Input: part model. Units: mm. Frame: model coordinates. Coordinates: 2 decimals unless noted, no trailing zeros. Order: outer loops, then holes, each group sorted by start corner. A loop starts at its lowest first (then second) coordinate and runs counter-clockwise, first axis right, second up. Notation, with made-up numbers: (-11, 17) -> (5, 17) arc R31 cw to (5, 44) -> close; hole circle Ø9 at (-18.5, 11). An arc over 180 degrees is marked (long way). Write each question's results on one line, items separated by ' | '.
```python
from build123d import *

# Parameters (mm, degrees)
SKETCH1_W                   = 80
SKETCH1_H                   = 130
SKETCH1_R                   = 3.5
BOSS_EXTRUDE1_DEPTH         = 8
DODANIE_WYCI_GNI_CIE1_DEPTH = 6
SZKIC2_W                    = 2
SZKIC2_H                    = 6
WYTNIJ_WYCI_GNI_CIE1_DEPTH  = 40


with BuildPart() as part:
    # Sketch1 → Boss-Extrude1 (new body)
    with BuildSketch(Plane(origin=(0, 0, 0), x_dir=(0, -1, 0), z_dir=(-1, 0, 0))):
        with Locations((-35, 60)):
            Rectangle(SKETCH1_W, SKETCH1_H)
        with Locations((-66, 116)):
            Circle(SKETCH1_R, mode=Mode.SUBTRACT)
        with Locations((-4, 116)):
            Circle(SKETCH1_R, mode=Mode.SUBTRACT)
    extrude(amount=-BOSS_EXTRUDE1_DEPTH)

    # Szkic1 → Dodanie-wyciągnięcie1 (add)
    with BuildSketch(Plane.ZY):
        Polygon((-3.873206623, 3.873206623), (3.197861189, -3.197861189), (6.733395095, 0.337672717), (-0.337672717, 7.408740528), align=None)
        Polygon((20.875530719, 28.621943964), (27.946598531, 21.550876152), (31.482132437, 25.086410058), (24.411064625, 32.15747787), align=None)
    extrude(amount=DODANIE_WYCI_GNI_CIE1_DEPTH)

    # Szkic2 → Wytnij-wyciągnięcie1 (cut)
    with BuildSketch(Plane(origin=(0, 0, 0), x_dir=(1, 0, 0), z_dir=(0, -0.707106781, -0.707106781))):
        with Locations((-3, -0.477541336)):
            Rectangle(SZKIC2_W, SZKIC2_H)
    extrude(amount=-WYTNIJ_WYCI_GNI_CIE1_DEPTH, mode=Mode.SUBTRACT)


solid = part.part
```
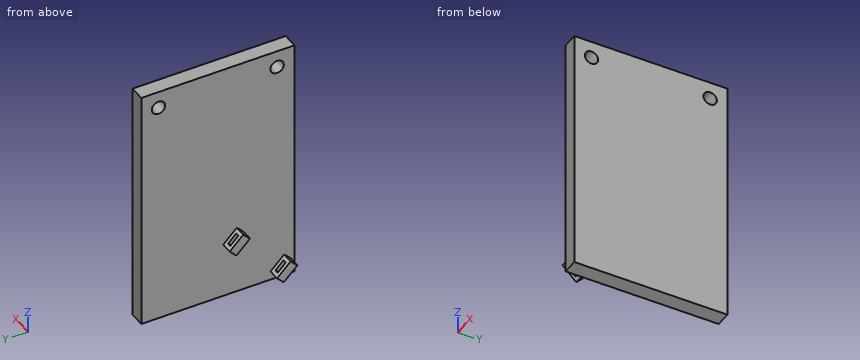
(1) Line query: line 1 along Z through (x, y) = (4, 66); line 2 along X through (y, z) = (29.5, 118.5); line 3 along Y through (x, z) = (3.75, 119). Output: solid intervals per line, ascending. Write a range as from..to.
Return value:
line 1: -5..112.5, 119.5..125 | line 2: 0..8 | line 3: -5..2.2, 5.8..64.2, 67.8..75
(2) Cut plane C-C, the plane z = 80. Return loops of the section in (x, y), plus the area to 3 significant figures.
Return value:
outline: (0, -5) -> (8, -5) -> (8, 75) -> (0, 75) -> close | area: 640 mm2
(3) Cut plane A-A, the plane y = 66. Return loops of the section in (x, z).
Return value:
outline: (0, -5) -> (8, -5) -> (8, 112.5) -> (0, 112.5) -> close; (0, 119.5) -> (8, 119.5) -> (8, 125) -> (0, 125) -> close
(4) Cut plane B-B, the plane z = 116. Return loops of the section in (x, y), plus the area to 3 significant figures.
Return value:
outline: (0, -5) -> (8, -5) -> (8, 0.5) -> (0, 0.5) -> close; (0, 7.5) -> (8, 7.5) -> (8, 62.5) -> (0, 62.5) -> close; (0, 69.5) -> (8, 69.5) -> (8, 75) -> (0, 75) -> close | area: 528 mm2
(5) Pin query (flat end, axial travel): P1, Ø10, axis at y = 52, z = 46, coming from the -X side; P2, Ø1, axis at x = -2, z = 73, coming from the -Y side. Return the tip coordinate at first contact, or that it passes through.
Return value:
P1: x = 0 | P2: through
